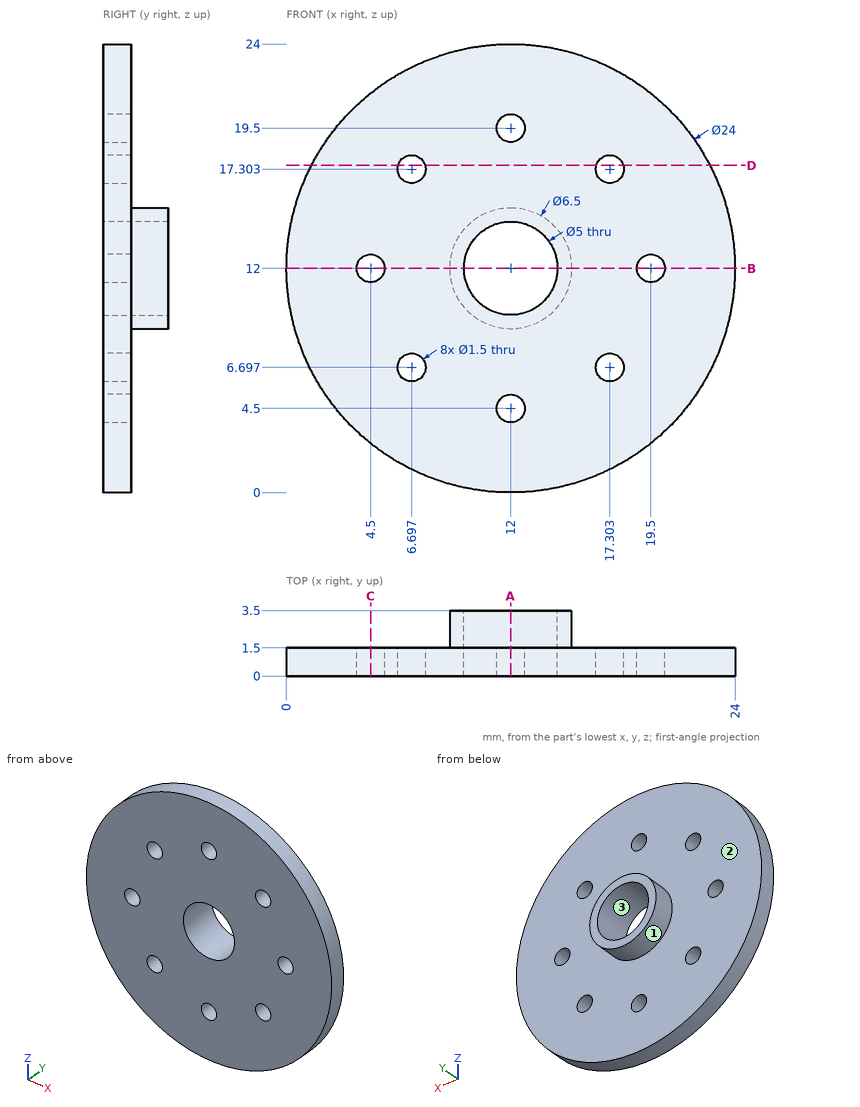
The figure shows three views and two pictorial views of one solid part (mm, origin at its lowest corner). Answer the questions. Round coordinates to 2 decimals unless told otherwise and drop trailing zeros. Loops run counter-clockwise (first coordinate to the right, second up) from the corner with the lowest first, then second, coordinate; pieces in that order, holes last. Notation, with made-up numbers: M 78,89.25 L 123,89.25 A15 cw 123,102.25 Z; hole C 10.5,49 d3. An arc over 180 degrees is marked long. Use CSV: the item, a comma, the result in double quotes.
Q1. Section B-B, the plane z = 12 is taken. Determine the outline of the cut face in (x, y), then the cut area to 3 significant figures.
Determined:
outline,"M 0,0 L 3.75,0 L 3.75,1.5 L 0,1.5 Z; M 5.25,0 L 9.5,0 L 9.5,3.5 L 8.75,3.5 L 8.75,1.5 L 5.25,1.5 Z; M 14.5,0 L 18.75,0 L 18.75,1.5 L 15.25,1.5 L 15.25,3.5 L 14.5,3.5 Z; M 20.25,0 L 24,0 L 24,1.5 L 20.25,1.5 Z"
area,"27.0 mm2"
Q2. The mould has two halves that part along X. Classify the marked faces 1, 2 and 3: pulls with the +X half, pulls with the -X half, needs draft (parallel to the pull), parting line crosses it, or undercut.
Determined:
face 1,"parting line crosses it"
face 2,"needs draft"
face 3,"undercut"
Q3. Consider L1, parallel to X at y = 0.3, z = 12; L2, parallel to Z at x = 12.5, y = 0.35; L3, parallel to Y at x = 1.75, z = 17.75. Determine where each line is inside the solid, lowest interval first.
Determined:
L1,"0 to 3.75, 5.25 to 9.5, 14.5 to 18.75, 20.25 to 24"
L2,"0.01 to 3.94, 5.06 to 9.55, 14.45 to 18.94, 20.06 to 23.99"
L3,"0 to 1.5"
Q4. Section C-C, the plane x = 4.5 is taken. Determine the outline of the cut face in (y, z).
Determined:
outline,"M 0,2.63 L 1.5,2.63 L 1.5,11.25 L 0,11.25 Z; M 0,12.75 L 1.5,12.75 L 1.5,21.37 L 0,21.37 Z"
Q5. Section D-D, the plane z = 17.5 is taken. Determine the outline of the cut face in (x, y) (1 decimal).
Determined:
outline,"M 1.3,0 L 6,0 L 6,1.5 L 1.3,1.5 Z; M 7.4,0 L 16.6,0 L 16.6,1.5 L 7.4,1.5 Z; M 18,0 L 22.7,0 L 22.7,1.5 L 18,1.5 Z"
Q6. Section A-A, the plane x = 12 is taken. Determine the outline of the cut face in (y, z), then the cut area to 3 significant figures.
Determined:
outline,"M 0,0 L 1.5,0 L 1.5,3.75 L 0,3.75 Z; M 0,5.25 L 1.5,5.25 L 1.5,8.75 L 3.5,8.75 L 3.5,9.5 L 0,9.5 Z; M 0,14.5 L 3.5,14.5 L 3.5,15.25 L 1.5,15.25 L 1.5,18.75 L 0,18.75 Z; M 0,20.25 L 1.5,20.25 L 1.5,24 L 0,24 Z"
area,"27.0 mm2"
Q7. This flat-tipped pin is pushed along its axis until it touches: pin 1 (5 mm diameter, centred on x = 2.5, z = 18, fed in from +Y). Where does it stop, or does it pass through?
Determined:
pin 1,"y = 1.5"
